Model file for the job. Use its own axes, mm. A direction names the side the tool comes from. Coordinates: 2 decimals unless noted, no trailing zeros. Loops run counter-clockwise (first coordinate to the right, second up) from the corner with the lowest first, then second, coordinate; pieces in that order, holes last.
from build123d import *

# Parameters (mm, degrees)
BOSS_EXTRUDE1_DEPTH = 3
CUT_EXTRUDE1_REACH  = 5
SKETCH2_W           = 20
SKETCH2_H           = 2.9


with BuildPart() as part:
    # Sketch1 → Boss-Extrude1 (new body)
    with BuildSketch(Plane(origin=(0, 0, 0), x_dir=(1, 0, 0), z_dir=(0, 1, 0))):
        with BuildLine():
            Line((-50, 30), (-21.914, 30))
            Line((-21.914, 30), (-21.914, 25))
            Line((-21.914, 25), (-19.214, 25))
            Line((-19.214, 25), (-19.214, 30))
            Line((-19.214, 30), (8.872, 30))
            ThreePointArc((8.872, 30), (14.965992065, 27.304879145), (18.013850136, 21.379427525))
            Line((18.013850136, 21.379427525), (13.013850136, 21.379427525))
            Line((13.013850136, 21.379427525), (13.013850136, 18.679427525))
            Line((13.013850136, 18.679427525), (18.013850136, 18.679427525))
            ThreePointArc((18.013850136, 18.679427525), (14.965992065, 12.753975906), (8.872, 10.058855051))
            Line((8.872, 10.058855051), (-19.214, 10.058855051))
            Line((-19.214, 10.058855051), (-19.214, 15.058855051))
            Line((-19.214, 15.058855051), (-21.914, 15.058855051))
            Line((-21.914, 15.058855051), (-21.914, 10.058855051))
            Line((-21.914, 10.058855051), (-50, 10.058855051))
            ThreePointArc((-50, 10.058855051), (-56.093992065, 12.753975906), (-59.141850136, 18.679427525))
            Line((-59.141850136, 18.679427525), (-54.141850136, 18.679427525))
            Line((-54.141850136, 18.679427525), (-54.141850136, 21.379427525))
            Line((-54.141850136, 21.379427525), (-59.141850136, 21.379427525))
            ThreePointArc((-59.141850136, 21.379427525), (-56.093992065, 27.304879145), (-50, 30))
        make_face()
    extrude(amount=BOSS_EXTRUDE1_DEPTH)

    # Sketch2 → Cut-Extrude1 (cut, up to next)
    with BuildSketch(Plane(origin=(0, 3, 0), x_dir=(1, 0, 0), z_dir=(0, 1, 0)), mode=Mode.PRIVATE) as cut_extrude1_sk1:
        with Locations((-35.957, 20.029427525)):
            Rectangle(SKETCH2_W, SKETCH2_H)
    cut_extrude1_tool1 = extrude(cut_extrude1_sk1.sketch, amount=-CUT_EXTRUDE1_REACH, mode=Mode.PRIVATE) & part.part
    add(cut_extrude1_tool1.solids().sort_by_distance((-35.957, 3, -20.029428))[0], mode=Mode.SUBTRACT)
    # Sketch2 → Cut-Extrude1 (cut, up to next)
    with BuildSketch(Plane(origin=(0, 3, 0), x_dir=(1, 0, 0), z_dir=(0, 1, 0)), mode=Mode.PRIVATE) as cut_extrude1_sk2:
        with Locations((-5.171, 20.029427525)):
            Rectangle(SKETCH2_W, SKETCH2_H)
    cut_extrude1_tool2 = extrude(cut_extrude1_sk2.sketch, amount=-CUT_EXTRUDE1_REACH, mode=Mode.PRIVATE) & part.part
    add(cut_extrude1_tool2.solids().sort_by_distance((-5.171, 3, -20.029428))[0], mode=Mode.SUBTRACT)


solid = part.part
Q1. Slice it at A-A (x = -7). List the corners of the cut face in (y, z), and give its area (3 significant figures).
Answers:
outline: (0, -30) - (3, -30) - (3, -21.48) - (0, -21.48) - close; (0, -18.58) - (3, -18.58) - (3, -10.06) - (0, -10.06) - close
area: 51.1 mm2
Q2. Which spindle directions (+Z, -Z, +X, -X, +Y, -Y) get a long thin tool onto all of the face, cutting with end or side? Do faces 4 (the flat face through (13.014, 1, -20)), 5 (the flat face through (-21.914, 1, -13)), 6 (the flat face through (-54.142, 1, -20)), 7 (the flat face through (4.829, 2, -20)), 8 (the flat face through (-19.214, 1, -27)). Say none if no direction does.
Answers:
face 4: +X, +Y, -Y
face 5: +Z, +Y, -Y
face 6: -X, +Y, -Y
face 7: +Y, -Y
face 8: -Z, +Y, -Y
Q3. Slice it at D-D (z = -23.75). List the corners of the cut face in (x, y), and give its area (3 significant figures).
Answers:
outline: (-58.52, 0) - (17.39, 0) - (17.39, 3) - (-58.52, 3) - close
area: 228 mm2
Q4. Slice it at C-C (z = -12). List the corners of the cut face in (x, y).
Answers:
outline: (-55.19, 0) - (-21.91, 0) - (-21.91, 3) - (-55.19, 3) - close; (-19.21, 0) - (14.07, 0) - (14.07, 3) - (-19.21, 3) - close
Q5. Mould opens along X. For faces 1 (the flat face through (-21.914, 1, -28)), 2 (the cylindrical face through (15.035, 1.479, -12.82)), 3 (the flat face through (16, 1, -21.379)) say: +X half, -X half, draft (parallel to the pull), parting line (faces both ways), or undercut.
Answers:
face 1: undercut
face 2: +X half
face 3: draft
Q6. Drill centre lines: line 1 (X direction, y = 0.3, z = -21.25); line 2 (Z direction, x = -13.5, y = 2.05); line 3 (X direction, y = 1.1, z = -28). Where is each one in solid material? Low to high.
Answers:
line 1: x = -54.14 to -45.96, -25.96 to -15.17, 4.83 to 13.01
line 2: z = -30 to -21.48, -18.58 to -10.06
line 3: x = -55.27 to -21.91, -19.21 to 14.14
Q7. Flat gauge pins, fed straight in: P1, Ø1.3, axis at y = 1.5, z = -20.5, coming from the +X side; P2, Ø0.9, axis at y = 2, z = -19.5, coming from the -X side; P3, Ø0.9, axis at x = -55.5, y = 2, coming from the -Z side. Where does each tip first touch, or does it go through?
Answers:
P1: stops at x = 13.01
P2: stops at x = -54.14
P3: stops at z = -28.16
Q8. Slice it at B-B (y = 0.9). List the corners of the cut face in (x, z).
Answers:
outline: (-59.14, -21.38) arc R10 ccw to (-50, -30) - (-21.91, -30) - (-21.91, -25) - (-19.21, -25) - (-19.21, -30) - (8.87, -30) arc R10 ccw to (18.01, -21.38) - (13.01, -21.38) - (13.01, -18.68) - (18.01, -18.68) arc R10 ccw to (8.87, -10.06) - (-19.21, -10.06) - (-19.21, -15.06) - (-21.91, -15.06) - (-21.91, -10.06) - (-50, -10.06) arc R10 ccw to (-59.14, -18.68) - (-54.14, -18.68) - (-54.14, -21.38) - close; hole (-45.96, -21.48) - (-25.96, -21.48) - (-25.96, -18.58) - (-45.96, -18.58) - close; hole (-15.17, -21.48) - (4.83, -21.48) - (4.83, -18.58) - (-15.17, -18.58) - close
